from build123d import *

# Parameters (mm, degrees)
F0_W     = 70.104
F0_H     = 70.104
F1_DEPTH = 450
F2_W     = 50
F2_H     = 370
F3_DEPTH = 10
F4_W     = 200
F4_H     = 300
F5_DEPTH = 19
F6_W     = 50
F6_H     = 3
F7_DEPTH = 254


with BuildPart() as f1:
    # F0 (on Top) → F1 (new body)
    with BuildSketch(Plane.XY):
        with BuildLine():
            Line((34.925, 38.1), (-34.925, 38.1))
            ThreePointArc((-34.925, 38.1), (-37.1700640303, 37.1700640303), (-38.1, 34.925))
            Line((-38.1, 34.925), (-38.1, -34.925))
            ThreePointArc((-38.1, -34.925), (-37.1700640303, -37.1700640303), (-34.925, -38.1))
            Line((-34.925, -38.1), (34.925, -38.1))
            ThreePointArc((34.925, -38.1), (37.1700640303, -37.1700640303), (38.1, -34.925))
            Line((38.1, -34.925), (38.1, 34.925))
            ThreePointArc((38.1, 34.925), (37.1700640303, 37.1700640303), (34.925, 38.1))
        make_face()
        Rectangle(F0_W, F0_H, mode=Mode.SUBTRACT)
    extrude(amount=-F1_DEPTH)

    # F2 (on face) → F3 (join)
    with BuildSketch(Plane(origin=(-38.1, 0, 0), x_dir=(0, -1, 0), z_dir=(-1, 0, 0))):
        with Locations((0, -265)):
            Rectangle(F2_W, F2_H)
    extrude(amount=F3_DEPTH)

    # F4 (on Top) → F5 (join)
    with BuildSketch(Plane.XY):
        Rectangle(F4_W, F4_H)
    extrude(amount=F5_DEPTH)

    # F6 (on face) → F7 (cut)
    with BuildSketch(Plane(origin=(-100, 0, 0), x_dir=(0, -1, 0), z_dir=(-1, 0, 0))):
        with Locations((125, 1.5)):
            Rectangle(F6_W, F6_H)
        with Locations((-125, 1.5)):
            Rectangle(F6_W, F6_H)
    extrude(amount=-F7_DEPTH, mode=Mode.SUBTRACT)


solid = f1.part
Geometry check sheet. Reference: the model listing, model coordinates, mm. A direction names the side the tool comes from. Coordinates: 2 decimals unless noted, no trailing zeros. Order: outer loops, then holes, each group sorted by start corner. A loop starts at its lowest first (then second) coordinate and runs counter-clockwise, first axis right, second up. Notation, with made-up numbers: (-23, -21) - (2, -21) arc R19 ccw to (2, 15) - close; hole circle Ø11 at (82, 19). An arc over 180 degrees is marked (long way). One line per item, written item: value.
(1) Sectioned sample at A-A (z = -52). Enter the section's corners in (x, y) (3 decimals).
Data:
outline: (-38.1, -34.925) arc R3.175 ccw to (-34.925, -38.1) - (34.925, -38.1) arc R3.175 ccw to (38.1, -34.925) - (38.1, 34.925) arc R3.175 ccw to (34.925, 38.1) - (-34.925, 38.1) arc R3.175 ccw to (-38.1, 34.925) - close; hole (-35.052, -35.052) - (35.052, -35.052) - (35.052, 35.052) - (-35.052, 35.052) - close
(2) Release check for a two-part mould opening along X. For faces 4 (the face through (-35.052, 0, -222)), 5 (the face through (-1, 150, 11)), 6 (the face through (-48.1, 0, -262)), 7 (the face through (38.1, 0, -222)) record: +X half, -X half, draft (parallel to the pull), parting line (faces both ways), or undercut.
Data:
face 4: undercut
face 5: draft
face 6: -X half
face 7: +X half
(3) Access from +Z, -Z, +X, -X, +Y, -Y to the whole of each face (thin tool, end or side, straight path). Record for faces 1 (the face through (0, 35.052, -222)), 2 (the face through (-43, 0, -80)), 3 (the face through (-1, -125, 3)).
Data:
face 1: -Z
face 2: -X, +Y, -Y
face 3: -Z, +X, -X, -Y
(4) Depth check by flat-ended pin: pin 1 Ø8 at (y, z) = (-22.5, -250.5) entering from +X; pin 2 Ø10 at (x, z) = (25, -48.5) entering from +Y; pin 3 Ø3 at (x, z) = (-9, -45) entering from -Y. Enter the tip coordinate at first touch or a pass-through.
Data:
pin 1: stops at x = 38.1
pin 2: stops at y = 38.1
pin 3: stops at y = -38.1
(5) Sectioned sample at B-B (y = 0.5). Enter the section's corners in (x, z), and give its area (3 significant figures).
Data:
outline: (-100, 0) - (-38.1, 0) - (-38.1, -80) - (-48.1, -80) - (-48.1, -450) - (-35.05, -450) - (-35.05, 0) - (35.05, 0) - (35.05, -450) - (38.1, -450) - (38.1, 0) - (100, 0) - (100, 19) - (-100, 19) - close
area: 10,200 mm^2
(6) Sectioned sample at C-C (x = 14). Enter the section's corners in (y, z), and give its area (3 significant figures).
Data:
outline: (-150, 3) - (-100, 3) - (-100, 0) - (-38.1, 0) - (-38.1, -450) - (-35.05, -450) - (-35.05, 0) - (35.05, 0) - (35.05, -450) - (38.1, -450) - (38.1, 0) - (100, 0) - (100, 3) - (150, 3) - (150, 19) - (-150, 19) - close
area: 8,140 mm^2
(7) Thickness scan on probe 1 along Y at (x, z) = (25, -234.5); probe 2 along X at (y, z) = (-1.5, -336.5). Record the ranges inside material, lowest first. Write a range as from..to.
Data:
probe 1: y = -38.1..-35.05, 35.05..38.1
probe 2: x = -48.1..-35.05, 35.05..38.1
(8) Sectioned sample at D-D (x = 75). Enter the section's corners in (y, z).
Data:
outline: (-150, 3) - (-100, 3) - (-100, 0) - (100, 0) - (100, 3) - (150, 3) - (150, 19) - (-150, 19) - close
